from build123d import *

# Parameters (mm, degrees)
SKETCH1_R          = 2.413
EXTRUDE1_DEPTH     = 13.0302
CHAMFER1_SIZE      = 0.889
SKETCH3_W          = 4.826
SKETCH3_H          = 1.27
CUT_EXTRUDE1_DEPTH = 1.27


with BuildPart() as part:
    # Sketch1 → Extrude1 (new body)
    with BuildSketch(Plane.XY):
        with Locations((6.35, 0)):
            Circle(SKETCH1_R)
    extrude(amount=EXTRUDE1_DEPTH)

    # Chamfer1
    chamfer1_edges = [part.edges().sort_by_distance(p)[0] for p in [
        (3.937, 0, 0),
    ]]
    chamfer(chamfer1_edges, length=CHAMFER1_SIZE)

    # Sketch3 → Cut-Extrude1 (cut)
    with BuildSketch(Plane.XY.offset(13.0302)):
        with Locations((6.35, 0)):
            Rectangle(SKETCH3_W, SKETCH3_H)
    extrude(amount=-CUT_EXTRUDE1_DEPTH, mode=Mode.SUBTRACT)

    # Sketch4 → Revolve3 (revolve)
    with BuildSketch(Plane(origin=(0, 0, 0), x_dir=(1, 0, 0), z_dir=(0, 1, 0))):
        with BuildLine():
            Line((6.35, 0.635), (6.35, -1.7526))
            ThreePointArc((6.35, -1.7526), (5.1562, -0.5588), (6.35, 0.635))
        make_face()
    revolve(axis=Axis((6.35, 0, -0.635), (0, 0, 1)))


solid = part.part
Input: part model. Units: mm. Frame: model coordinates. A direction names the side the tool comes from. Coordinates: 2 decimals unless noted, no trailing zeros. Order: outer loops, then holes, each group sorted by start corner. A loop starts at its lowest first (then second) coordinate and runs counter-clockwise, first axis right, second up. Notation, with made-up numbers: M -37.75,34.25 L 14.25,34.25 A22 cw 14.25,65.25 Z; hole C 81.25,41.25 d11. An arc over 180 degrees is marked long. Answer in a Markdown table with one row per item.
(1) Draft query along Y for faces 1 (the flat face through (6, -0.635, 12)), 2 (the cylindrical face through (8.652, 0.725, 6.875)), 3 (the flat face through (6, 1, 13.03)). Return one class per face: pulls with the +Y half, pulls with the -Y half, needs draft (parallel to the pull), parting line crosses it, or undercut.
Numbers:
| item | result |
|---|---|
| face 1 | undercut |
| face 2 | parting line crosses it |
| face 3 | needs draft |
(2) Access query for faces 4 (the flat face through (6, -1, 13.03)), 5 (the flat face through (6, 0.635, 12)), 6 (the flat face through (5, 0, 0)). Directions: +Z, -Z, +X, -X, +Y, -Y. A direction counts if a zero-diameter tool reaches every point of the face in a straight line with its end or side. Return the directions, or none.
Numbers:
| item | result |
|---|---|
| face 4 | +Z, +X, -X, +Y, -Y |
| face 5 | +Z, +X, -X |
| face 6 | -Z |
(3) Material intervals for line 1 (Z direction, x = 5.25, y = 0.8); line 2 (Y direction, x = 8.15, z = 11.25); line 3 (X direction, y = 1.3, z = 8.75), sorted ascending. Write a range as [from, to].
Numbers:
| item | result |
|---|---|
| line 1 | z = [0, 13.03] |
| line 2 | y = [-1.61, 1.61] |
| line 3 | x = [4.32, 8.38] |
(4) Contact query for flat-ended pins moving along their axis: pin 1 Ø0.6 at (x, z) = (5, 12.5) entering from -Y; pin 2 Ø1.5 at (y, z) = (1, 3.5) entering from -X; pin 3 Ø1 at (x, z) = (7, 12.5) entering from +Y. Output: stop coordinate, or through.
Numbers:
| item | result |
|---|---|
| pin 1 | stops at y = -2.17 |
| pin 2 | stops at x = 3.95 |
| pin 3 | stops at y = 2.41 |
(5) Section query A-A, the plane x = 6.35. Output: boundary loops of the cut face in (y, z) (3 decimals).
Numbers:
| item | result |
|---|---|
| outline | M -2.413,0.889 L -1.524,0 L -1.055,0 A1.194 ccw 1.055,0 L 1.524,0 L 2.413,0.889 L 2.413,13.03 L 0.635,13.03 L 0.635,11.76 L -0.635,11.76 L -0.635,13.03 L -2.413,13.03 Z |
(6) Section query B-B, the plane y = 0. Output: boundary loops of the cut face in (x, z).
Numbers:
| item | result |
|---|---|
| outline | M 3.94,0.89 L 4.83,0 L 5.3,0 A1.19 ccw 7.4,0 L 7.87,0 L 8.76,0.89 L 8.76,11.76 L 3.94,11.76 Z |
(7) Section query C-C, the plane z = 3.75. Output: boundary loops of the cut face in (x, y).
Numbers:
| item | result |
|---|---|
| outline | C 6.35,0 d4.83 |
